```python
from build123d import *

# Parameters (mm, degrees)
BOSS_EXTRUDE1_DEPTH = 23
CUT_EXTRUDE1_DEPTH  = 52.51698749
SKETCH3_R           = 1.625
SKETCH3_R_2         = 5
CUT_EXTRUDE2_DEPTH  = 52.980765673


with BuildPart() as part:
    # Sketch1 → Boss-Extrude1 (new, symmetric)
    with BuildSketch(Plane.XY):
        Polygon((0, 0), (-30, 0), (-30, 38), (-27, 38), (-27, 3), (0, 3), align=None)
    extrude(amount=BOSS_EXTRUDE1_DEPTH, both=True)

    # Sketch2 → Cut-Extrude1 (cut, through all)
    with BuildSketch(Plane(origin=(0, 3, 0), x_dir=(1, 0, 0), z_dir=(0, 1, 0))):
        with BuildLine():
            Line((-6.5, -16), (-20.5, -16))
            ThreePointArc((-20.5, -16), (-22.5, -14), (-20.5, -12))
            Line((-20.5, -12), (-6.5, -12))
            ThreePointArc((-6.5, -12), (-4.5, -14), (-6.5, -16))
        make_face()
        with BuildLine():
            Line((-6.5, 16), (-20.5, 16))
            ThreePointArc((-20.5, 16), (-22.5, 14), (-20.5, 12))
            Line((-20.5, 12), (-6.5, 12))
            ThreePointArc((-6.5, 12), (-4.5, 14), (-6.5, 16))
        make_face()
    extrude(amount=-CUT_EXTRUDE1_DEPTH, mode=Mode.SUBTRACT)

    # Sketch3 → Cut-Extrude2 (cut, through all)
    with BuildSketch(Plane(origin=(-27, 0, 0), x_dir=(0, 0, -1), z_dir=(1, 0, 0))):
        with Locations((-16.45, 31.11)):
            Circle(SKETCH3_R)
        with Locations((-8, 22)):
            Circle(SKETCH3_R_2)
        with Locations((-16.45, 12.91)):
            Circle(SKETCH3_R)
        with Locations((8, 22)):
            Circle(SKETCH3_R_2)
        with Locations((16.45, 31.11)):
            Circle(SKETCH3_R)
        with Locations((16.45, 12.91)):
            Circle(SKETCH3_R)
    extrude(amount=-CUT_EXTRUDE2_DEPTH, mode=Mode.SUBTRACT)


solid = part.part
```
Part model, mm, in its own coordinate system. A direction names the side the tool comes from. Round coordinates to 2 decimals unless told otherwise and drop trailing zeros. Loops run counter-clockwise (first coordinate to the right, second up) from the corner with the lowest first, then second, coordinate; pieces in that order, holes last. Notation, with made-up numbers: (-7, -19.5) -> (40, -19.5) arc R20 ccw to (40, -11.5) -> close; hole circle Ø11 at (-24.5, 11.5). An arc over 180 degrees is marked (long way). Use CSV: the item, a comma, the result in double quotes. Start each with the question number.
1) Pull direction Y, two halves, no side cores. Call faces 4 (the cylindrical face through (-28.48, 30.12, 17.74)), 5 (the cylindrical face through (-22.5, 1.5, 14)), 6 (the flat face through (-29, 38, 0)): +Y half, -Y half, draft (parallel to the pull), parting line (faces both ways), or undercut.
2) Drop flat-ended pins along their axis: P1, Ø5, axis at x = -3.5, z = 13, coming from the +Y side; P2, Ø11.5, axis at y = 22, z = -8, coming from the +X side. Give the stop position or say it passes through.
3) Cut at A-A, the plane y = 31.11. Write the cut outline in (x, z) (3 decimals), plus the area to 4 significant figures.
4) Which spindle directions (+Z, -Z, +X, -X, +Y, -Y) get a long thin tool onto all of the face, cutting with end or side? Do faces 1 (the cylindrical face through (-28.48, 30.12, -15.16)), 2 (the flat face through (-27, 21, 0)), 3 (the flat face through (-14, 2, -12)). Say none if no direction does.
5) Cut at D-D, the plane z = 1. Write the cut outline in (x, y), plus the area to 3 significant figures.
6) Wall check: L1, parallel to Z at x = -27.5, y = 31; L2, parallel to Y at x = -28.6, z = -16.45 (3 decimals); L3, parallel to Z at x = -20, y = 2. Give the ranges that are in metal, low to high. Write a range as [from, to].
7) Cut at B-B, the plane z = 14. Write the cut outline in (x, y).
8) Cut at C-C, the plane x = -8.25. Write the cut outline in (y, z), plus the area to 3 significant figures.
Determined:
1,face 4,"undercut"
1,face 5,"draft"
1,face 6,"+Y half"
2,P1,"stops at y = 3"
2,P2,"stops at x = -27"
3,outline,"(-30, -23) -> (-27, -23) -> (-27, -18.075) -> (-30, -18.075) -> close; (-30, -14.825) -> (-27, -14.825) -> (-27, 14.825) -> (-30, 14.825) -> close; (-30, 18.075) -> (-27, 18.075) -> (-27, 23) -> (-30, 23) -> close"
3,area,"118.5 mm2"
4,face 1,"+X, -X"
4,face 2,"+Z, -Z, +X, +Y"
4,face 3,"+Y, -Y"
5,outline,"(-30, 0) -> (0, 0) -> (0, 3) -> (-27, 3) -> (-27, 38) -> (-30, 38) -> close"
5,area,"195 mm2"
6,L1,"z = [-23, -18.07], [-14.83, 14.83], [18.07, 23]"
6,L2,"y = [0, 11.285], [14.535, 29.485], [32.735, 38]"
6,L3,"z = [-23, -16], [-12, 12], [16, 23]"
7,outline,"(-30, 0) -> (-22.5, 0) -> (-22.5, 3) -> (-27, 3) -> (-27, 38) -> (-30, 38) -> close; (-4.5, 0) -> (0, 0) -> (0, 3) -> (-4.5, 3) -> close"
8,outline,"(0, -23) -> (3, -23) -> (3, -16) -> (0, -16) -> close; (0, -12) -> (3, -12) -> (3, 12) -> (0, 12) -> close; (0, 16) -> (3, 16) -> (3, 23) -> (0, 23) -> close"
8,area,"114 mm2"
